Geometry: final body of the model. Coordinates: model frame, mm. A direction names the side the tool comes from. Round coordinates to 2 decimals unless told otherwise and drop trailing zeros. Order: outer loops, then holes, each group sorted by start corner. A loop starts at its lowest first (then second) coordinate and runs counter-clockwise, first axis right, second up. Notation, with made-up numbers: M 13.5,22.5 L 60.5,22.5 A27 ccw 60.5,61.5 Z; hole C 6,30.5 d1. An arc over 180 degrees is marked long. Return JSON: item names as keys, results as strings. Group by question number.
Q1. Cut plane B-B on y = 15. Output: boundary loops of the cut face in (x, z), and give its area (3 significant figures).
Q2. Mould query, pull axis Z, two halves, no side actions, for faces 4 (the face through (14, 40, 12)), 5 (the face through (10.09, -18.48, 28.38)), 6 (the face through (18, 10, -1)). Classes: released by +Z, released by -Z, zero draft, split by the parting line, or undercut.
Q3. Cut plane D-D on z = 26. Output: boundary loops of the cut face in (x, y).
Q4. Contact query for flat-ended pins moving along their axis: pin 1 (12 mm diameter, centred on y = -9.5, z = 11.5, fed in from +X); pin 2 (4.5 mm diameter, centred on x = 4, y = 15, fed in from +Z); pin 3 (10 mm diameter, centred on y = -7.5, z = 16, fed in from +X); pin 4 (12.5 mm diameter, centred on x = 15.5, y = 31.5, fed in from -Z). Output: stop coordinate, or through.
Q5. Cut plane C-C on x = 23.5. Output: boundary loops of the cut face in (y, z), and give its area (3 significant figures).
Q6. Access query for faces 1 (the face through (21.6, -17, 4.1)), 2 (the face through (26.446, 38.521, 2.433)), 3 (the face through (20.614, 10, 5)). Directions: +Z, -Z, +X, -X, +Y, -Y. A direction counts if a zero-diameter tool reaches every point of the face in a straight line with its end or side. Return the directions, or none.
Q7. Cut plane A-A on x = 33. Output: boundary loops of the cut face in (y, z), and give its area (3 significant figures).
Q8. Ray query, probe 1 along Y at (x, z) = (4, -0.25); probe 2 along Z at (x, y) = (14, -15.5); probe 3 along Z at (x, y) = (12.5, 13.5). Return the intervals inside material, ascending.
```python
from build123d import *

# Parameters (mm, degrees)
SKETCH_1_W          = 30
SKETCH_1_H          = 20
SKETCH_1_R          = 2
EXTRUDE_2_DEPTH     = 1
SKETCH_3_W          = 2
SKETCH_3_H          = 20
EXTRUDE_4_DEPTH     = 6
SKETCH_4_R          = 2
CUT_EXTRUDE_1_DEPTH = 6
EXTRUDE_START       = -17
SKETCH_8_W          = 10.614335182
SKETCH_8_H          = 6.998118079
EXTRUDE_6_DEPTH     = 54
EXTRUDE_START_2     = 17
SKETCH_2_R          = 2
EXTRUDE_7_DEPTH     = 3
EXTRUDE_START_3     = -40
SKETCH_2_2_R        = 2
EXTRUDE_8_DEPTH     = 3


with BuildPart() as part:
    # 草图1 → 凸台-拉伸2 (new, symmetric)
    with BuildSketch(Plane.XY):
        with Locations((15, 10)):
            Rectangle(SKETCH_1_W, SKETCH_1_H)
        with Locations((4, 15)):
            Circle(SKETCH_1_R, mode=Mode.SUBTRACT)
        with Locations((4, 5)):
            Circle(SKETCH_1_R, mode=Mode.SUBTRACT)
    extrude(amount=EXTRUDE_2_DEPTH, both=True)

    # 草图3 → 凸台-拉伸4 (add)
    with BuildSketch(Plane(origin=(30, 0, 0), x_dir=(0, 0, -1), z_dir=(1, 0, 0))):
        with Locations((0, 10)):
            Rectangle(SKETCH_3_W, SKETCH_3_H)
    extrude(amount=EXTRUDE_4_DEPTH)

    # 草图4 → 切除-拉伸1 (cut)
    with BuildSketch(Plane.XY.offset(1)):
        with Locations((33, 15)):
            Circle(SKETCH_4_R)
        with Locations((33, 5)):
            Circle(SKETCH_4_R)
    extrude(amount=-CUT_EXTRUDE_1_DEPTH, mode=Mode.SUBTRACT)

    # 草图8 → 凸台-拉伸6 (add)
    with BuildSketch(Plane(origin=(0, 0, 0), x_dir=(1, 0, 0), z_dir=(0, 1, 0)).offset(EXTRUDE_START)):
        with Locations((15.307167591, -4.49905904)):
            Rectangle(SKETCH_8_W, SKETCH_8_H)
    extrude(amount=EXTRUDE_6_DEPTH)

    # 草图2 → 凸台-拉伸7 (add)
    with BuildSketch(Plane.XZ.offset(EXTRUDE_START_2)):
        with BuildLine():
            Line((10, 1), (21.263932023, 1))
            ThreePointArc((21.263932023, 1), (26.462284118, 2.525792445), (22, 5.598076211))
            Line((22, 5.598076211), (11.5, 23.784609691))
            ThreePointArc((11.5, 23.784609691), (9.223542865, 29.280463381), (10, 23.382685902))
            Line((10, 23.382685902), (10, 3))
            Line((10, 3), (10, 1))
        make_face()
        with Locations(Location((23.5, 3, 0), (0, 0, 270))):
            Circle(SKETCH_2_R, mode=Mode.SUBTRACT)
        with Locations(Location((10, 26.382685902, 0), (0, 0, 270))):
            Circle(SKETCH_2_R, mode=Mode.SUBTRACT)
    extrude(amount=EXTRUDE_7_DEPTH)

    # 草图2<2> → 凸台-拉伸8 (add)
    with BuildSketch(Plane.XZ.offset(EXTRUDE_START_3)):
        with BuildLine():
            Line((10, 1), (21.263932023, 1))
            ThreePointArc((21.263932023, 1), (26.462284118, 2.525792445), (22, 5.598076211))
            Line((22, 5.598076211), (11.5, 23.784609691))
            ThreePointArc((11.5, 23.784609691), (9.223542865, 29.280463381), (10, 23.382685902))
            Line((10, 23.382685902), (10, 3))
            Line((10, 3), (10, 1))
        make_face()
        with Locations(Location((23.5, 3, 0), (0, 0, 270))):
            Circle(SKETCH_2_2_R, mode=Mode.SUBTRACT)
        with Locations(Location((10, 26.382685902, 0), (0, 0, 270))):
            Circle(SKETCH_2_2_R, mode=Mode.SUBTRACT)
    extrude(amount=EXTRUDE_8_DEPTH)


solid = part.part
```
Result sheet:
{
 "1": {"outline": "M 0,-1 L 2,-1 L 2,1 L 0,1 Z; M 6,-1 L 31,-1 L 31,1 L 20.61,1 L 20.61,8 L 10,8 L 10,1 L 6,1 Z; M 35,-1 L 36,-1 L 36,1 L 35,1 Z", "area": "130 mm²"},
 "2": {"face 4": "zero draft", "face 5": "undercut", "face 6": "released by -Z"},
 "3": {"outline": "M 7.02,-20 L 8.04,-20 L 8.04,-17 L 7.02,-17 Z; M 7.02,37 L 8.04,37 L 8.04,40 L 7.02,40 Z; M 11.96,-20 L 12.98,-20 L 12.98,-17 L 11.96,-17 Z; M 11.96,37 L 12.98,37 L 12.98,40 L 11.96,40 Z"},
 "4": {"pin 1": "stops at x = 20.61", "pin 2": "stops at z = 1", "pin 3": "passes through", "pin 4": "stops at z = 1"},
 "5": {"outline": "M -20,0 L -17,0 L -17,1 L -20,1 Z; M -20,5 L -17,5 L -17,6 L -20,6 Z; M 0,-1 L 20,-1 L 20,1 L 0,1 Z; M 37,0 L 40,0 L 40,1 L 37,1 Z; M 37,5 L 40,5 L 40,6 L 37,6 Z", "area": "52.0 mm²"},
 "6": {"face 1": "+Z, -Z, +X", "face 2": "+Y", "face 3": "+Z, +X"},
 "7": {"outline": "M 0,-1 L 3,-1 L 3,1 L 0,1 Z; M 7,-1 L 13,-1 L 13,1 L 7,1 Z; M 17,-1 L 20,-1 L 20,1 L 17,1 Z", "area": "24.0 mm²"},
 "8": {"probe 1": "y = 0 to 3, 7 to 13, 17 to 20", "probe 2": "z = 1 to 8", "probe 3": "z = -1 to 8"}
}
